Work out the finished part from the listing and answer in its coordinate system (mm). A direction names the side the tool comes from. Coordinates: 2 decimals unless noted, no trailing zeros. Write each loop counter-clockwise with the first axis right and the second up, starting at its lowest first coordinate (ties: lowest second). Pieces come first, ordered by that corner, then holes. Notation, with made-up numbers: (-27, 67) - (9, 67) arc R22 cw to (9, 88) - close; hole circle Ø5 at (31, 29). An arc over 180 degrees is marked (long way). Use one line per item in the form item = value. Start each with the question number.
Item 1: For faces 5 (the flat face through (-16, 1, 0)), 6 (the flat face through (10.19, -7.08, -3.45)), 7 (the flat face through (0, 40, -10)), 8 (the cylindrical face through (-15, 23, -14)), 9 (the flat face through (-0.322, 32.664, -14.504)), determine the directions among +Z, -Z, +X, -X, +Y, -Y from which every point of the face is accessible in a straight line to the end or side of a thin tool.
Item 2: A cutting plane is placed at B-B (y = -2.5). Write down the section's boundary in (x, z).
Item 3: Consider probe 1 along Y at (x, z) = (-1, -10) (3 decimals); probe 2 along Y at (x, z) = (9, -8); probe 3 along X at (y, z) = (-6.5, -18.75). Determine where each line is inside the solid, lowest interval first.
Item 4: A cutting plane is placed at D-D (x = 19). Give the number of separate pieces and of enclosed holes in the cut face, then the cut area to 3 significant figures.
Item 5: A cutting plane is placed at A-A (z = -10). Write down the section's boundary in (x, y) (3 decimals).
Item 6: A cutting plane is placed at C-C (z = -18.5). Write down the section's boundary in (x, y).
Item 7: Given pin 1 (2 mm diameter, centred on x = 2.5, y = 9.5, fed in from -Z); pin 2 (2 mm diameter, centred on x = -15, y = -12, fed in from -Z), each flat-ended and moving along its own axis, determine where each tip first touches the part or whether it passes through.
Item 8: Determine the mould class of faces 1 (the cylindrical face through (-0.3, -31.3, -5.8)), 2 (the flat face through (0, -40, -10)), 3 (the flat face through (-23, 1, -10)), 4 (the cylindrical face through (-11, 11.06, -3.45)) for opening direction Y: released by +Y, released by -Y, zero draft, split by the parting line, or undercut.
Solid Edge part; units mm, degrees
sketch "Sketch1" plane through (0, 0, 0) normal (0, 0, 1) x (1, 0, 0)
  line L0 (-23, -40) -> (23, -40)
  line L1 (23, -40) -> (23, 40)
  line L2 (23, 40) -> (-23, 40)
  line L3 (-23, 40) -> (-23, -40)
extrude "Protrusion1" add sketch "Sketch1" against normal blind 20
sketch "Sketch2" plane through (-23, 0, -10) normal (-1, 0, 0) x (0, -1, 0)
  circle A0 centre (31.175, 0) radius 4.2
  circle A1 centre (-31.175, 0) radius 4.2
  dimension "D1" = 31.175
extrude "Cutout1" cut sketch "Sketch2" against normal through all
sketch "Sketch3" plane through (-23, 0, -10) normal (-1, 0, 0) x (0, -1, 0)
  line L0 (31.175, 0) -> (34.1962, -2.9176)
  line L1 (34.1962, -2.9176) -> (31.175, -6.0461)
  line L2 (31.175, -6.0461) -> (28.1538, -2.9176)
  line L3 (28.1538, -2.9176) -> (31.175, 0)
  line L4 (-31.175, 0) -> (-28.1538, -2.9176)
  line L5 (-28.1538, -2.9176) -> (-31.175, -6.0461)
  line L6 (-31.175, -6.0461) -> (-34.1962, -2.9176)
  line L7 (-34.1962, -2.9176) -> (-31.175, 0)
extrude "Cutout2" cut sketch "Sketch3" against normal through all
sketch "Sketch4" plane through (0, 0, -20) normal (0, 0, -1) x (0, -1, 0)
  line L0 (-24, -17) -> (24, -17)
  line L1 (24, -17) -> (24, 17)
  line L2 (24, 17) -> (-24, 17)
  line L3 (-24, 17) -> (-24, -17)
  dimension "D1" = 24
  dimension "D2" = 24
extrude "Cutout3" cut sketch "Sketch4" against normal up to vertex (13 mm away)
sketch "Sketch5" plane through (0, 0, 0) normal (0, 0, 1) x (1, 0, 0)
  arc A0 (-9.3209, -6.2097) -> (-9.3209, 6.2097) centre (0, 0) cw
  line L0 (-11.0309, 7.9196) -> (-9.3209, 6.2097)
  arc A1 (-11.0309, 7.9196) -> (-7.9196, 11.0309) centre (-9.4752, 9.4752) cw
  line L1 (-7.9196, 11.0309) -> (-6.2097, 9.3209)
  arc A2 (-6.2097, 9.3209) -> (6.2097, 9.3209) centre (0, 0) cw
  line L2 (7.9196, 11.0309) -> (6.2097, 9.3209)
  line L3 (11.0309, 7.9196) -> (9.3209, 6.2097)
  line L4 (11.0309, -7.9196) -> (9.3209, -6.2097)
  arc A3 (11.0309, -7.9196) -> (7.9196, -11.0309) centre (9.4752, -9.4752) cw
  line L5 (7.9196, -11.0309) -> (6.2097, -9.3209)
  arc A4 (6.2097, -9.3209) -> (-6.2097, -9.3209) centre (0, 0) cw
  line L6 (-7.9196, -11.0309) -> (-6.2097, -9.3209)
  arc A5 (-7.9196, -11.0309) -> (-11.0309, -7.9196) centre (-9.4752, -9.4752) cw
  line L7 (-11.0309, -7.9196) -> (-9.3209, -6.2097)
  arc A6 (7.9196, 11.0309) -> (11.0309, 7.9196) centre (9.4752, 9.4752) cw
  arc A7 (9.3209, 6.2097) -> (9.3209, -6.2097) centre (0, 0) cw
extrude "Cutout4" cut sketch "Sketch5" against normal through all
fillet "Round_1" radius 5 4 edges at (-17, 24, -13.5) (-17, -24, -13.5) (17, -24, -13.5) (17, 24, -13.5)
fillet "Round_2" radius 2 8 edges at (0, -24, -7) (-15.5355, -22.5355, -7) (-17, 0, -7) (-15.5355, 22.5355, -7) (0, 24, -7) (15.5355, 22.5355, -7) (17, 0, -7) (15.5355, -22.5355, -7)
Answer:
q1.face_5 = +Z, +X, -X, +Y, -Y
q1.face_6 = +Z, -Z
q1.face_7 = +Z, -Z, +X, -X, +Y
q1.face_8 = -Z
q1.face_9 = +X, -X
q2.outline = (-23, -20) - (-17, -20) - (-17, -9) arc R2 cw to (-15, -7) - (-10.92, -7) - (-10.92, 0) - (-23, 0) - close; (10.92, -7) - (15, -7) arc R2 cw to (17, -9) - (17, -20) - (23, -20) - (23, 0) - (10.92, 0) - close
q3.probe_1 = -40 to -35.375, -26.975 to -24, 24 to 26.975, 35.375 to 40
q3.probe_2 = -40 to -34.87, -27.48 to -23.73, 23.73 to 27.48, 34.87 to 40
q3.probe_3 = -23 to -17, 17 to 23
q4.separate_pieces = 1
q4.enclosed_holes = 2
q4.area = 1,480 mm²
q5.outline = (-23, -40) - (23, -40) - (23, -35.375) - (-23, -35.375) - close; (-23, -26.975) - (23, -26.975) - (23, 26.975) - (-23, 26.975) - close; (-23, 35.375) - (23, 35.375) - (23, 40) - (-23, 40) - close; hole (-17, -19) arc R5 ccw to (-12, -24) - (12, -24) arc R5 ccw to (17, -19) - (17, 19) arc R5 ccw to (12, 24) - (-12, 24) arc R5 ccw to (-17, 19) - close
q6.outline = (-23, -40) - (23, -40) - (23, 40) - (-23, 40) - close; hole (-17, -19) arc R5 ccw to (-12, -24) - (12, -24) arc R5 ccw to (17, -19) - (17, 19) arc R5 ccw to (12, 24) - (-12, 24) arc R5 ccw to (-17, 19) - close
q7.pin_1 = through
q7.pin_2 = -7.27
q8.face_1 = undercut
q8.face_2 = released by -Y
q8.face_3 = zero draft
q8.face_4 = undercut
